Design review of the part built by this model. Coordinates are the model's own, in mm. A direction names the side the tool comes from. Round coordinates to 2 decimals unless told otherwise and drop trailing zeros. Write each loop counter-clockwise with the first axis right and the second up, starting at its lowest first coordinate (ties: lowest second). Pieces come first, ordered by that corner, then holes.
Autodesk Fusion 360 part; units mm, degrees
sketch "Sketch1" plane through (0, 0, 0) normal (1, 0, 0) x (0, 1, 0)
  line L0 (0, 0) -> (0, -99.0463) construction
  line L1 (-30.4057, -88.0396) -> (0, -88.0396)
  arc A0 (-37.6553, -37.4456) -> (-22.2115, -8.1006) centre (-43.2405, -15.7698) ccw
  arc A1 (-37.6553, -37.4456) -> (-30.4057, -88.0396) centre (-31.2401, -62.3428) ccw
  arc A2 (0, 23.6426) -> (-22.2115, -8.1006) centre (0, 0) ccw
  arc A3 (22.2115, -8.1006) -> (0, 23.6426) centre (0, 0) ccw
  line L2 (30.4057, -88.0396) -> (0, -88.0396)
  arc A4 (30.4057, -88.0396) -> (37.6553, -37.4456) centre (31.2401, -62.3428) ccw
  arc A5 (22.2115, -8.1006) -> (37.6553, -37.4456) centre (43.2405, -15.7698) ccw
extrude "Extrude1" add sketch "Sketch1" along normal blind 8.398
sketch "Sketch2" plane through (8.398, 0, 0) normal (1, 0, 0) x (0, 1, 0)
  circle A0 centre (-33.7553, -79.2573) radius 3.7955
extrude "Extrude2" add sketch "Sketch2" along normal blind 10
fillet "Fillet1" radius 2.082 1 edges at (18.398, -37.294, -80.6298)
sketch "Sketch3" plane through (8.398, 0, 0) normal (1, 0, 0) x (0, 1, 0)
  circle A0 centre (-33.7553, -79.2573) radius 3.7955
  arc A1 (22.2115, -8.1006) -> (-22.2115, -8.1006) centre (0, 0) ccw
  arc A2 (-37.6553, -37.4456) -> (-22.2115, -8.1006) centre (-43.2405, -15.7698) ccw
  arc A3 (-37.6553, -37.4456) -> (-30.4057, -88.0396) centre (-31.2401, -62.3428) ccw
  line L0 (-30.4057, -88.0396) -> (30.4057, -88.0396)
  arc A4 (30.4057, -88.0396) -> (37.6553, -37.4456) centre (31.2401, -62.3428) ccw
  arc A5 (22.2115, -8.1006) -> (37.6553, -37.4456) centre (43.2405, -15.7698) ccw
  arc A6 (14.1938, -5.1765) -> (-14.1938, -5.1765) centre (0, 0) ccw
  arc A7 (-35.5258, -45.7099) -> (-14.1938, -5.1765) centre (-43.2405, -15.7698) ccw
  arc A8 (-35.5258, -45.7099) -> (-30.5582, -79.5054) centre (-31.2401, -62.3428) ccw
  line L1 (-30.5582, -79.5054) -> (30.5582, -79.5054)
  arc A9 (30.5582, -79.5054) -> (35.5258, -45.7099) centre (31.2401, -62.3428) ccw
  arc A10 (14.1938, -5.1765) -> (35.5258, -45.7099) centre (43.2405, -15.7698) ccw
  dimension "d6" = 8.5343
1) For line 1 along X through (y, z) = (-16, -22); line 2 along Z through (x, y) = (6.75, 43); line 3 along Y through (x, z) = (6, -57), list the stretches that pass through material, from the lowest coordinate up.
2) For P1, Ø1, axis at x = 5, z = -36, coming from the +Y side; P2, Ø5, axis at x = 8.5, y = -12.5, coming from the -Z side; P3, Ø10, axis at y = -12, z = 9, coming from the +X side, all flat-tipped, find the tip position at first contact; note any pin that passes through.
3) The part is to be moulded in two halves that separate along Z. For faces 3 (the face through (18.398, -34, -79)), 4 (the face through (4.14, -23.31, -25.96)), 5 (the face through (4.14, -56.61, -66.51)), say which applies: pulls with the +Z half, pulls with the -Z half, needs draft (parallel to the pull), parting line crosses it, or undercut.
4) Add section D-D on x = 14.5. State the section outline as (y, z) points.
5) Add section A-A on x = 2. State the section outline as (y, z) points, and give its area (3 significant figures).
6) Add section B-B on y = -48.5. State the section outline as (x, z) points.
7) Add section C-C on z = -73. State the section outline as (x, y) points, and give its area (3 significant figures).
8) For faces 1 (the face through (12.302, -34.578, -75.552)), 2 (the face through (0, -1, -44)), list the 3-axis set-ups (+Z, -Z, +X, -X, +Y, -Y) from which the entire face can be reached by the end or side of a thin tool; tool diameter is ignored.
Computed:
1. line 1: x = 0 to 8.4
1. line 2: z = -85.21 to -39.48
1. line 3: y = -56.39 to 56.39
2. P1: stops at y = 34.8
2. P2: stops at z = -88.04
2. P3: stops at x = 8.4
3. face 3: needs draft
3. face 4: undercut
3. face 5: parting line crosses it
4. outline: circle Ø7.59 at (-33.76, -79.26)
5. outline: (-37.66, -37.45) arc R25.71 ccw to (-30.41, -88.04) - (30.41, -88.04) arc R25.71 ccw to (37.66, -37.45) arc R22.38 cw to (22.21, -8.1) arc R23.64 ccw to (0, 23.64) arc R23.64 ccw to (-22.21, -8.1) arc R22.38 cw to start
5. area: 7,900 mm2
6. outline: (0, -81.4) - (8.4, -81.4) - (8.4, -43.29) - (0, -43.29) - close
7. outline: (0, -54.64) - (8.4, -54.64) - (8.4, 54.64) - (0, 54.64) - close
7. area: 918 mm2
8. face 1: +X
8. face 2: +Z, -Z, -X, +Y, -Y
